For this review, take the finished solid that the model builds, in its own axes (mm). A direction names the side the tool comes from. Give positions to 0.01 mm unless a question says otherwise; leave off trailing zeros. Order: outer loops, then holes, each group sorted by start corner. A loop starts at its lowest first (then second) coordinate and runs counter-clockwise, first axis right, second up. Notation, with made-up numbers: (-5.5, 61) - (24.5, 61) arc R29 cw to (24.5, 82) - close; hole circle Ø10 at (23, 35.5). An arc over 180 degrees is marked (long way). Use a Markdown table: item, result. Add a question column.
1) Clearance check with flat-ended pins moving along their axes: P1, Ø0.9, axis at x = -0.5, y = -0.5, coming from the +Z side; P2, Ø0.6, axis at x = -0.5, z = 0, coming from the +Y side; P3, Ø1, axis at y = -12.5, z = 0, coming from the +X side. State where each tip first meets the part, or that it passes through.
2) Wall thickness on L1, parallel to Y at x = 0.5, z = 0; L2, parallel to Y at x = -2, z = -1.25; L3, parallel to Z at x = -0.5, y = -1: over which ranges is each line inside the solid? List them lowest first.
3) We need section B-B on y = -4.25. Write out the cut boundary in (x, z), then the cut area to 3 significant figures.
4) We need section A-A on x = 0. Write out the cut boundary in (y, z).
5) Mouldability with a two-part tool opening along X and no side actions: class faces 1 (the face through (-0.87, -0.54, 0.49)), 2 (the face through (-0.45, -8.68, 1.43)), 3 (the face through (0, -1.1, 0)), 4 (the face through (0, -16, 0)) as released by +X, released by -X, zero draft, split by the parting line, or undercut.
6) Machinability: for faces 5 (the face through (1, 0, -1)), 6 (the face through (-0.86, -0.54, -0.51)), which of the approach directions +Z, -Z, +X, -X, +Y, -Y give a long, thin tool a straight path to every point of the face, cutting with its end or side? Answer none if there is none.
```python
from build123d import *

# Parameters (mm, degrees)
ESQUISSE_TETE_R         = 3.36
EXTRUSION_TETE_DEPTH    = 1.86
ENL_V_MAT_EXTRU_1_DEPTH = 1.1
ESQUISSE_CORPS_R        = 1.5
EXTRUSION_CORPS_DEPTH   = 14.14
CHANFREIN_SIZE          = 0.3


with BuildPart() as part:
    # Esquisse TETE → Extrusion TETE (new body)
    with BuildSketch(Plane(origin=(0, 0, 0), x_dir=(1, 0, 0), z_dir=(0, 1, 0))):
        with Locations(Location((0, 0, 0), (0, 0, 270))):
            Circle(ESQUISSE_TETE_R)
    extrude(amount=-EXTRUSION_TETE_DEPTH)

    # Esquisse1 → Enlèv. mat.-Extru.1 (cut)
    with BuildSketch(Plane(origin=(0, 0, 0), x_dir=(1, 0, 0), z_dir=(0, 1, 0))):
        Polygon((0.577350269, -1), (1.154700538, 0), (0.577350269, 1), (-0.577350269, 1), (-1.154700538, 0), (-0.577350269, -1), align=None)
    extrude(amount=-ENL_V_MAT_EXTRU_1_DEPTH, mode=Mode.SUBTRACT)

    # Esquisse CORPS → Extrusion CORPS (add)
    with BuildSketch(Plane.XZ.offset(1.86)):
        with Locations(Location((0, 0, 0), (0, 0, 90))):
            Circle(ESQUISSE_CORPS_R)
    extrude(amount=EXTRUSION_CORPS_DEPTH)

    # Esquisse FRAISAGE → Enlèvement de matière-Révolution1 (revolve, cut)
    with BuildSketch(Plane(origin=(0, 0, 0), x_dir=(0, 0, -1), z_dir=(1, 0, 0))):
        Polygon((-1.5, -1.86), (-3.1, -0.26), (-3.1, 0), (-3.36, 0), (-3.36, -1.86), align=None)
    revolve(axis=Axis((0, 0, 0), (0, -1, 0)), mode=Mode.SUBTRACT)

    # Chanfrein
    chanfrein_edges = [part.edges().sort_by_distance(p)[0] for p in [
        (0, -16, -1.5),
    ]]
    chamfer(chanfrein_edges, length=CHANFREIN_SIZE)


solid = part.part
```
Checked values:
| question | item | result |
|---|---|---|
| 1 | P1 | z = 3.1 |
| 1 | P2 | y = -1.1 |
| 1 | P3 | x = 1.5 |
| 2 | L1 | -16 to -1.1 |
| 2 | L2 | -1 to 0 |
| 2 | L3 | -2.31 to -1, 1 to 2.31 |
| 3 | outline | circle Ø3 at (0, 0) |
| 3 | area | 7.07 mm² |
| 4 | outline | (-16, -1.2) - (-15.7, -1.5) - (-1.86, -1.5) - (-0.26, -3.1) - (0, -3.1) - (0, -1) - (-1.1, -1) - (-1.1, 1) - (0, 1) - (0, 3.1) - (-0.26, 3.1) - (-1.86, 1.5) - (-15.7, 1.5) - (-16, 1.2) - close |
| 5 | face 1 | undercut |
| 5 | face 2 | split by the parting line |
| 5 | face 3 | undercut |
| 5 | face 4 | zero draft |
| 6 | face 5 | +Z, -Z, +X, -X, +Y |
| 6 | face 6 | +Y |
